```python
from build123d import *

# Parameters (mm, degrees)
SKETCH047_R          = 20.955
PAD005_DEPTH         = 33.02
SKETCH048_R          = 20.955
PAD006_DEPTH         = 25.4
SKETCH050_R          = 19.304
POCKET005_DEPTH      = 33.021
POCKET005_DEPTH_BACK = 33.021
SKETCH049_R          = 19.304
POCKET006_DEPTH      = 25.401
SKETCH051_R          = 22.86
SKETCH051_R_2        = 14.605
PAD007_DEPTH         = 9.906
SKETCH052_R          = 22.86
SKETCH052_R_2        = 14.605
PAD008_DEPTH         = 9.906
SKETCH053_R          = 22.86
SKETCH053_R_2        = 14.605
PAD009_DEPTH         = 9.906


with BuildPart() as part:
    # Sketch047 → Pad005 (new body, symmetric)
    with BuildSketch(Plane.YZ):
        Circle(SKETCH047_R)
    extrude(amount=PAD005_DEPTH, both=True)

    # Sketch048 → Pad006 (join)
    with BuildSketch(Plane.XZ):
        Circle(SKETCH048_R)
    extrude(amount=PAD006_DEPTH)

    # Sketch050 → Pocket005 (cut, two sides)
    with BuildSketch(Plane.YZ) as pocket005_sk:
        Circle(SKETCH050_R)
    extrude(amount=-POCKET005_DEPTH, mode=Mode.SUBTRACT)
    extrude(pocket005_sk.sketch, amount=POCKET005_DEPTH_BACK, mode=Mode.SUBTRACT)

    # Sketch049 → Pocket006 (cut, through all)
    with BuildSketch(Plane.XZ):
        Circle(SKETCH049_R)
    extrude(amount=POCKET006_DEPTH, mode=Mode.SUBTRACT)

    # Sketch051 (on Face6 of Pocket006) → Pad007 (join)
    with BuildSketch(Plane(origin=(0, -25.4, 0), x_dir=(0, 0, -1), z_dir=(0, -1, 0))):
        Circle(SKETCH051_R)
        Circle(SKETCH051_R_2, mode=Mode.SUBTRACT)
    extrude(amount=PAD007_DEPTH)

    # Sketch052 (on Face8 of Pad007) → Pad008 (join)
    with BuildSketch(Plane(origin=(-33.02, 0, 0), x_dir=(0, 1, 0), z_dir=(-1, 0, 0))):
        Circle(SKETCH052_R)
        Circle(SKETCH052_R_2, mode=Mode.SUBTRACT)
    extrude(amount=PAD008_DEPTH)

    # Sketch053 (on Face6 of Pad008) → Pad009 (join)
    with BuildSketch(Plane.YZ.offset(33.02)):
        Circle(SKETCH053_R)
        Circle(SKETCH053_R_2, mode=Mode.SUBTRACT)
    extrude(amount=PAD009_DEPTH)


with BuildPart() as part_1:
    # Body013 placement: moved
    add(part.part.moved(Location((-381, 0, 0))))


solid = part_1.part
```
Verification items for the finished model (mm, model axes). A direction names the side the tool comes from. Round coordinates to 2 decimals unless told otherwise and drop trailing zeros. Write each loop counter-clockwise with the first axis right and the second up, starting at its lowest first coordinate (ties: lowest second). Pieces come first, ordered by that corner, then holes. Notation, with made-up numbers: (40.25, 39.5) -> (74.25, 39.5) arc R21 cw to (74.25, 53.5) -> close; hole circle Ø6 at (43.5, -38). An arc over 180 degrees is marked (long way). Write each question's results on one line, items separated by ' | '. Start each with the question number.
1. Cross-section at B-B (y = 10). Enter the section's corners in (x, z) (3 decimals), then the cut area to 3 significant figures.
2. Cross-section at A-A (z = -17). Enter the section's corners in (x, y).
3. Cross-section at C-C (x = -364). Enter the section's corners in (y, z) (3 decimals), then the cut area to 3 significant figures.
4. Draft check along X on faces 5 (the flat face through (-423.926, 0, 15)), 6 (the cylindrical face through (-358.335, -30.284, 2.976)), 7 (the flat face through (-368, -25.4, -7)), 8 (the cylindrical face through (-418.904, 21.804, -6.867)). Enter one of: +X half, -X half, draft (parallel to the pull), parting line (faces both ways), or undercut.
5. Cross-section at D-D (z = 0). Count the separate pieces of the cut face and the enclosed holes in it, then the cut area to 3 significant figures.
6. Material ranges on probe 1 along Y at (x, z) = (-416.5, 0) (3 decimals); probe 2 along Z at (x, y) = (-381, -7.5) (3 decimals), recorded low to high. Write a range as from..to.
7. Set-up check for faces 1 (the flat face through (-347.98, 19, -10)), 2 (the cylindrical face through (-395.258, -30.284, 3.166)), 3 (the cylindrical face through (-343.096, 21.804, 6.867)), 4 (the flat face through (-338.074, 0, -15)): record each of +Z, -Z, +X, -X, +Y, -Y from which the full face is reachable in a straight line by a thin tool's end or side.
8. Depth check by flat-ended pin: P1, Ø1, axis at x = -366, z = -16.5, coming from the +Y side; P2, Ø23.5, axis at x = -381, z = 0, coming from the -Y side; P3, Ø19.5, axis at x = -372, z = -2, coming from the +Y side (3 decimals); P4, Ø17.5, axis at y = 0, z = 0, coming from the -X side. Enter the tip coordinate at first touch or a pass-through.
Solutions:
1) outline: (-423.926, -20.557) -> (-414.02, -20.557) -> (-414.02, -18.415) -> (-347.98, -18.415) -> (-347.98, -20.557) -> (-338.074, -20.557) -> (-338.074, -10.645) -> (-347.98, -10.645) -> (-347.98, -16.512) -> (-414.02, -16.512) -> (-414.02, -10.645) -> (-423.926, -10.645) -> close; (-423.926, 10.645) -> (-414.02, 10.645) -> (-414.02, 16.512) -> (-347.98, 16.512) -> (-347.98, 10.645) -> (-338.074, 10.645) -> (-338.074, 20.557) -> (-347.98, 20.557) -> (-347.98, 18.415) -> (-414.02, 18.415) -> (-414.02, 20.557) -> (-423.926, 20.557) -> close | area: 644 mm2
2) outline: (-423.93, -15.28) -> (-414.02, -15.28) -> (-414.02, -12.25) -> (-393.25, -12.25) -> (-393.25, -25.4) -> (-396.28, -25.4) -> (-396.28, -35.31) -> (-365.72, -35.31) -> (-365.72, -25.4) -> (-368.75, -25.4) -> (-368.75, -12.25) -> (-347.98, -12.25) -> (-347.98, -15.28) -> (-338.07, -15.28) -> (-338.07, 15.28) -> (-347.98, 15.28) -> (-347.98, 12.25) -> (-414.02, 12.25) -> (-414.02, 15.28) -> (-423.93, 15.28) -> close; hole (-414.02, -9.15) -> (-390.15, -9.15) -> (-390.15, -25.4) -> (-371.85, -25.4) -> (-371.85, -9.15) -> (-347.98, -9.15) -> (-347.98, 9.15) -> (-414.02, 9.15) -> close
3) outline: (-35.306, -15.283) -> (-25.4, -15.283) -> (-25.4, -12.252) -> (-17, -12.252) arc R20.955 ccw (long way) to (-17, 12.252) -> (-25.4, 12.252) -> (-25.4, 15.283) -> (-35.306, 15.283) -> close; hole (-25.4, -9.146) -> (-17, -9.146) arc R19.304 ccw (long way) to (-17, 9.146) -> (-25.4, 9.146) -> close | area: 526 mm2
4) face 5: -X half | face 6: parting line | face 7: undercut | face 8: draft
5) separate pieces: 3 | enclosed holes: 0 | area: 660 mm2
6) probe 1: y = -22.86..-14.605, 14.605..22.86 | probe 2: z = -20.955..-19.304, 19.304..20.955
7) face 1: none | face 2: -Y | face 3: +X | face 4: +Z, -Z, +X, +Y, -Y
8) P1: stops at y = 13.53 | P2: stops at y = 15.32 | P3: stops at y = 20.955 | P4: passes through
